from build123d import *

# Parameters (mm, degrees)
F0_W     = 25.4
F0_H     = 25.4
F0_W_2   = 19.05
F0_H_2   = 19.05
F1_DEPTH = 127
F2_R     = 2.54


with BuildPart() as f1:
    # F0 (on Front) → F1 (new body)
    with BuildSketch(Plane.XZ):
        Rectangle(F0_W, F0_H)
        Rectangle(F0_W_2, F0_H_2, mode=Mode.SUBTRACT)
    extrude(amount=F1_DEPTH)

    # F2
    f2_edges = [f1.edges().sort_by_distance(p)[0] for p in [
        (-12.7, -63.5, -12.7),
        (12.7, -63.5, -12.7),
        (-12.7, -63.5, 12.7),
        (12.7, -63.5, 12.7),
    ]]
    fillet(f2_edges, radius=F2_R)


solid = f1.part
Here's how the part is built. I have some questions about the finished solid (model axes, mm). A direction names the side the tool comes from. Round coordinates to 2 decimals unless told otherwise and drop trailing zeros. Order: outer loops, then holes, each group sorted by start corner. A loop starts at its lowest first (then second) coordinate and runs counter-clockwise, first axis right, second up. Notation, with made-up numbers: M 75.25,64.25 L 114.25,64.25 A33 ccw 114.25,96.25 Z; hole C 46,-7 d11. An arc over 180 degrees is marked long. Return JSON: item names as keys, results as strings. Group by question number.
1. On a 3-axis mill with a long thin cutter (end or side, diameter ignored), from which of +Z, -Z, +X, -X, +Y, -Y can I reach the whole of each face in a straight line? I mean faces 4 (the face through (0, -63, -9.525)), 5 (the face through (0, -63, 12.7)). Say none if no direction works.
2. If we section it at C-C on y = -117: List the corners of the cut face in (x, z) for me (3 decimals).
3. If we section it at B-B on x = -5.5: List the corners of the cut face in (y, z) for me (3 decimals), then the cut area to 3 significant figures.
4. If we section it at A-A on z = 1: List the corners of the cut face in (x, y) for me (3 decimals).
5. Please list where these lines run through material, in increasing order: probe 1 along Z at (x, y) = (-5, -81.5) (3 decimals); probe 2 along X at (y, z) = (-9.5, 10.25).
6. If we mould it in two halves opening along Z, with no side actions, what happens to faces 1 (the face through (-11.976, -64.389, 11.936)), 2 (the face through (-9.525, -63, 0)), 3 (the face through (11, 0, 0))? For each: pulls with the +Z half, pulls with the -Z half, needs draft (parallel to the pull), parting line crosses it, or undercut.
Reply:
{
 "1": {"face 4": "+Y, -Y", "face 5": "+Z, +X, -X, +Y, -Y"},
 "2": {"outline": "M -12.7,-10.16 A2.54 ccw -10.16,-12.7 L 10.16,-12.7 A2.54 ccw 12.7,-10.16 L 12.7,10.16 A2.54 ccw 10.16,12.7 L -10.16,12.7 A2.54 ccw -12.7,10.16 Z; hole M -9.525,-9.525 L 9.525,-9.525 L 9.525,9.525 L -9.525,9.525 Z"},
 "3": {"outline": "M -127,-12.7 L 0,-12.7 L 0,-9.525 L -127,-9.525 Z; M -127,9.525 L 0,9.525 L 0,12.7 L -127,12.7 Z", "area": "806 mm^2"},
 "4": {"outline": "M -12.7,-127 L -9.525,-127 L -9.525,0 L -12.7,0 Z; M 9.525,-127 L 12.7,-127 L 12.7,0 L 9.525,0 Z"},
 "5": {"probe 1": "-12.7 to -9.525, 9.525 to 12.7", "probe 2": "-12.7 to 12.7"},
 "6": {"face 1": "pulls with the +Z half", "face 2": "undercut", "face 3": "needs draft"}
}
